Verification items for the finished model (mm, model axes). Coordinates: 2 decimals unless noted, no trailing zeros. Order: outer loops, then holes, each group sorted by start corner. A loop starts at its lowest first (then second) coordinate and runs counter-clockwise, first axis right, second up. Notation, with made-up numbers: M 13.5,21.5 L 67.5,21.5 A33 ccw 67.5,50.5 Z; hole C 82,19 d10. An arc over 180 degrees is marked long. Return JSON: item names as keys, results as strings.
```python
from build123d import *

# Parameters (mm, degrees)
SKETCH2_W           = 4.7625
SKETCH2_H           = 4.7625
BOSS_EXTRUDE1_DEPTH = 4.7625


with BuildPart() as part:
    # Sketch2 → Boss-Extrude1 (new body)
    with BuildSketch(Plane.XY):
        with Locations((-2.38125, -96.67875)):
            Rectangle(SKETCH2_W, SKETCH2_H)
        with Locations((-2.38125, -4.92125)):
            Rectangle(SKETCH2_W, SKETCH2_H)
        Polygon((5.08, 0), (0, 0), (0, -2.54), (0, -7.3025), (0, -94.2975), (0, -99.06), (0, -101.6), (5.08, -101.6), (5.08, -96.8375), (12.7, -96.8375), (12.7, -101.6), (46.0375, -101.6), (46.0375, -96.8375), (53.6575, -96.8375), (53.6575, -101.6), (58.7375, -101.6), (58.7375, -88.9), (53.975, -88.9), (53.975, -81.28), (58.7375, -81.28), (58.7375, -20.32), (53.975, -20.32), (53.975, -12.7), (58.7375, -12.7), (58.7375, 0), (53.6575, 0), (53.6575, -4.7625), (46.0375, -4.7625), (46.0375, 0), (12.7, 0), (12.7, -4.7625), (5.08, -4.7625), align=None)
    extrude(amount=BOSS_EXTRUDE1_DEPTH)


solid = part.part
```
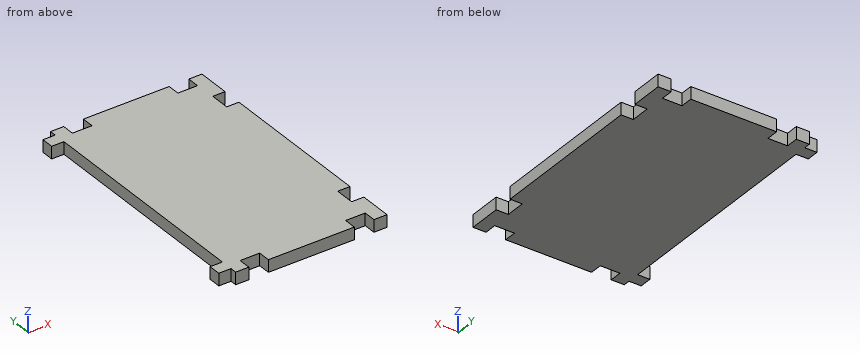
Q1. Cross-section at A-A, the plane x = 8.5. Record the boundary of the cut face in (y, z), and give its area (3 significant figures).
Values:
{"outline": "M -96.84,0 L -4.76,0 L -4.76,4.76 L -96.84,4.76 Z", "area": "439 mm^2"}
Q2. Material ranges on line 1 along X through (y, z) = (-60.5, 2.2); line 2 along Y through (x, z) = (49, 2.2); line 3 along X through (y, z) = (-83, 1.2) (3 decimals), recorded low to high.
Values:
{"line 1": "0 to 58.74", "line 2": "-96.84 to -4.76", "line 3": "0 to 53.975"}
Q3. Cross-section at B-B, the plane y = -84.5. Record the boundary of the cut face in (x, z) (1 decimal).
Values:
{"outline": "M 0,0 L 54,0 L 54,4.8 L 0,4.8 Z"}
Q4. Go/stop test with flat-tipped pins: pin 1 (1.4 mm diameter, centred on x = 49, z = 2, fed in from -Y); pin 2 (1 mm diameter, centred on y = -45, z = 3.5, fed in from -X); pin 3 (2.5 mm diameter, centred on y = -85, z = 3, fed in from +X) (3 decimals); pin 4 (2.5 mm diameter, centred on x = 57.5, z = 2, fed in from +Y). Record where each tip stops, or that it passes through.
Values:
{"pin 1": "y = -96.84", "pin 2": "x = 0", "pin 3": "x = 53.975", "pin 4": "y = 0"}
